```python
from build123d import *

# Parameters (mm, degrees)
F0_R     = 3.81
F1_DEPTH = 6.35
F2_R     = 1.27
F3_R     = 1.27
F4_DEPTH = 25.4


with BuildPart() as f1:
    # F0 (on Right) → F1 (new body)
    with BuildSketch(Plane.YZ):
        Circle(F0_R)
    extrude(amount=F1_DEPTH)

    # F2
    f2_edges = [f1.edges().sort_by_distance(p)[0] for p in [
        (6.35, -3.81, 0),
        (0, -3.81, 0),
    ]]
    fillet(f2_edges, radius=F2_R)

    # F3 (on face) → F4 (cut)
    with BuildSketch(Plane.YZ.offset(6.35)):
        Circle(F3_R)
    extrude(amount=-F4_DEPTH, mode=Mode.SUBTRACT)


solid = f1.part
```
Model file for the job. Use its own axes, mm. Give positions to 0.01 mm unless a question says otherwise; leave off trailing zeros. Loops run counter-clockwise (first coordinate to the right, second up) from the corner with the lowest first, then second, coordinate; pieces in that order, holes last. Notation, with made-up numbers: (-15.5, 55.25) - (9.5, 55.25) arc R12 cw to (9.5, 71.25) - close; hole circle Ø11 at (76.25, 24). An arc over 180 degrees is marked (long way). One line per item, written item: value. Start each with the question number.
1. Probe L1, parallel to Z at x = 5, y = 0; L2, parallel to Y at x = 3.25, z = -0.75; L3, parallel to Y at x = 6, z = 2. List the from-to ranges inside material, lowest first. Write a range as from..to.
2. Pin check, flat tip, straight feed: pin 1 (1 mm diameter, centred on x = 4, y = -2.5, fed in from +Z). Stop position of the tip, or through.
3. Slice it at C-C (x = 4.25). List the corners of the cut face in (y, z).
4. Pull direction Z, two halves, no side cores. Call faces 1 (the cylindrical face through (3.15, -0.83, -3.72)), 2 (the cylindrical face through (3.22, -0.17, 1.26)), 3 (the flat face through (6.35, 1.1, -1.1)): pulls with the +Z half, pulls with the -Z half, needs draft (parallel to the pull), parting line crosses it, or undercut.
5. Slice it at D-D (x = 1). List the corners of the cut face in (y, z), plus the area to 3 significant figures.
6. Slice it at A-A (z = 0). List the corners of the cut face in (x, y), plus the area to 3 significant figures.
Solution:
1. L1: z = -3.81..-1.27, 1.27..3.81
1. L2: y = -3.74..-1.02, 1.02..3.74
1. L3: y = -2.77..2.77
2. pin 1: stops at z = 3.24
3. outline: circle Ø7.62 at (0, 0); hole circle Ø2.54 at (0, 0)
4. face 1: parting line crosses it
4. face 2: undercut
4. face 3: needs draft
5. outline: circle Ø7.56 at (0, 0); hole circle Ø2.54 at (0, 0)
5. area: 39.8 mm^2
6. outline: (0, -2.54) arc R1.27 ccw to (1.27, -3.81) - (5.08, -3.81) arc R1.27 ccw to (6.35, -2.54) - (6.35, -1.27) - (0, -1.27) - close; (0, 1.27) - (6.35, 1.27) - (6.35, 2.54) arc R1.27 ccw to (5.08, 3.81) - (1.27, 3.81) arc R1.27 ccw to (0, 2.54) - close
6. area: 30.9 mm^2
